Read the model definition and answer for the solid it produces. Units are mm, in the model's axes. Face numbers are marked on the shaded views. A direction names the side the tool comes from. Coordinates: 2 decimals unless noted, no trailing zeros. Loops run counter-clockwise (first coordinate to the right, second up) from the corner with the lowest first, then second, coordinate; pieces in that order, holes last.
Q1. Flat-ended cylindrical pins translate along their axes: P1, Ø5, axis at y = 14.5, z = -1, coming from the +X side; P2, Ø1.5, axis at x = -4.5, y = 10, coming from the -Z side; P3, Ø3, axis at y = 15.5, z = -11.5, coming from the -X side; P4, Ø10, axis at x = -3.5, y = 11.5, coming from the +Z side. Find the tip coordinate at first contact, or state that the pin passes through.
Q2. Straight lines are drawn through the part: line 1 (X direction, y = 2.6, z = -16); line 2 (Y direction, x = -4.5, z = -4.5); line 3 (Y direction, x = 4.25, z = -10). For each, find the intervals that lie inside material, in ascending order.
Q3. The mould has two halves that part along X. Classify the marked faces 4, 5, 6 and 7: pulls with the +X half, pulls with the -X half, needs draft (parallel to the pull), parting line crosses it, or undercut.
Q4. Section A-A (z = -16) is taken. Give the vertices of the cut face in (x, y), then the cut area to 3 significant figures.
Q5. Section B-B (y = 18.5) is taken. Give the vertices of the cut face in (x, z).
Q6. Which of the six approach directions +Z, -Z, +X, -X, +Y, -Y give full straight-line access (tool end or side, diameter ignored) to the marked faces 1, 2 and 3?
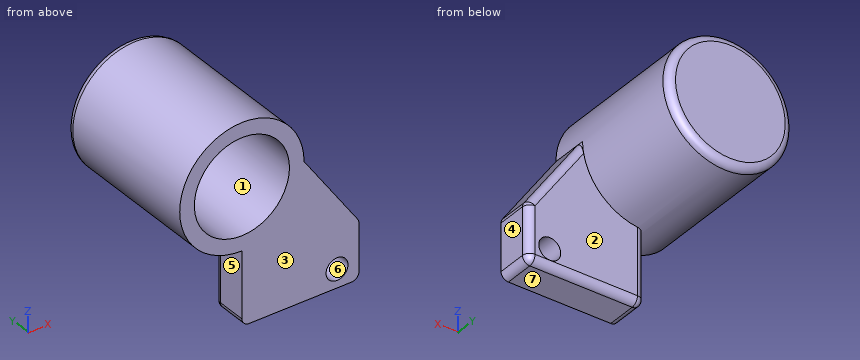
from build123d import *

# Parameters (mm, degrees)
SALIENTE_EXTRUIR1_START = -5
CROQUIS2_R              = 1.5
SALIENTE_EXTRUIR1_DEPTH = 5
REDONDEO1_R             = 1


with BuildPart() as part:
    # Croquis1 → Revolución1 (revolve)
    with BuildSketch(Plane.XY, mode=Mode.PRIVATE) as revoluci_n1_sk:
        Polygon((0, 19), (-6.5, 19), (-6.5, 0), (-8.5, 0), (-8.5, 21), (0, 21), align=None)
    revolve(revoluci_n1_sk.sketch.rotate(Axis((0, 0, 0), (0, 1, 0)), 270), axis=Axis((0, 0, 0), (0, 1, 0)))

    # Croquis2 → Saliente-Extruir1 (add)
    with BuildSketch(Plane.XZ.offset(SALIENTE_EXTRUIR1_START)):
        with BuildLine():
            Line((10, -18.5), (16, -18.5))
            Line((16, -18.5), (16, -10.75))
            Line((16, -10.75), (8.5, 0))
            ThreePointArc((8.5, 0), (6.01040764, -6.01040764), (0, -8.5))
            Line((0, -8.5), (0, -18.5))
            Line((0, -18.5), (10, -18.5))
        make_face()
        with Locations(Location((13, -16, 0), (0, 0, 270))):
            Circle(CROQUIS2_R, mode=Mode.SUBTRACT)
    extrude(amount=SALIENTE_EXTRUIR1_DEPTH)

    # Redondeo1
    # the kernel refuses this fillet: 1 mm, written as the material it takes off along each edge
    with BuildSketch(Plane(origin=(15, 4, -11.064363564), x_dir=(0.8201269543011832, 0, 0.5721815960240815), z_dir=(0, 1, 0))) as redondeo1_piece_1_section:
        Polygon((0, 0), (REDONDEO1_R, 0), (REDONDEO1_R, REDONDEO1_R * 0.314363563856), (REDONDEO1_R * 0.820126954301, REDONDEO1_R * 0.572181596024), align=None)
    redondeo1_piece_1 = extrude(amount=REDONDEO1_R, mode=Mode.PRIVATE)
    redondeo1_piece_1 = redondeo1_piece_1 - Plane(origin=(15, 4, -11.064363564), x_dir=(-0.9539724719039809, 0, -0.29989418608804086), z_dir=(0, 1, 0)) * Sphere(REDONDEO1_R, mode=Mode.PRIVATE)
    add(redondeo1_piece_1, mode=Mode.SUBTRACT)
    with BuildSketch(Plane(origin=(15, 4, -17.5), x_dir=(1, 0, 0), z_dir=(0, 0, -1))) as redondeo1_piece_2_section:
        Polygon((0, 0), (REDONDEO1_R, 0), (REDONDEO1_R, -REDONDEO1_R), (0, -REDONDEO1_R), align=None)
    redondeo1_piece_2 = extrude(amount=REDONDEO1_R, mode=Mode.PRIVATE)
    redondeo1_piece_2 = redondeo1_piece_2 - Plane(origin=(15, 4, -17.5), x_dir=(-0.7071067811865475, -0.7071067811865475, 0), z_dir=(0, 0, -1)) * Sphere(REDONDEO1_R, mode=Mode.PRIVATE)
    add(redondeo1_piece_2, mode=Mode.SUBTRACT)
    with BuildSketch(Plane(origin=(1, 4, -17.5), x_dir=(-1, 0, 0), z_dir=(0, 0, -1))) as redondeo1_piece_3_section:
        Polygon((0, 0), (REDONDEO1_R, 0), (REDONDEO1_R, REDONDEO1_R), (0, REDONDEO1_R), align=None)
    redondeo1_piece_3 = extrude(amount=REDONDEO1_R, mode=Mode.PRIVATE)
    redondeo1_piece_3 = redondeo1_piece_3 - Plane(origin=(1, 4, -17.5), x_dir=(0.7071067811865475, -0.7071067811865475, 0), z_dir=(0, 0, -1)) * Sphere(REDONDEO1_R, mode=Mode.PRIVATE)
    add(redondeo1_piece_3, mode=Mode.SUBTRACT)
    with BuildSketch(Plane(origin=(15.820126954, 5, -10.492181968), x_dir=(-0.8201269543011831, 0, -0.5721815960240815), z_dir=(-0.5721815960240815, 0, 0.8201269543011832))) as redondeo1_piece_4_section:
        with BuildLine():
            CenterArc((REDONDEO1_R, REDONDEO1_R), REDONDEO1_R, 180, 90)
            Line((0, REDONDEO1_R), (0, 0))
            Line((0, 0), (REDONDEO1_R, 0))
        make_face()
    redondeo1_piece_4 = extrude(amount=15.293363165, mode=Mode.PRIVATE)
    redondeo1_piece_4 = redondeo1_piece_4 - Plane(origin=(0, 4.770801137, 0), x_dir=(0, 0, -1), z_dir=(0, 1, 0)) * Cylinder(8.5, 35, mode=Mode.PRIVATE)
    add(redondeo1_piece_4, mode=Mode.SUBTRACT)
    with BuildSketch(Plane(origin=(16, 5, -17.5), x_dir=(-1, 0, 0), z_dir=(0, 0, 1))) as redondeo1_piece_5:
        with BuildLine():
            CenterArc((REDONDEO1_R, REDONDEO1_R), REDONDEO1_R, 180, 90)
            Line((0, REDONDEO1_R), (0, 0))
            Line((0, 0), (REDONDEO1_R, 0))
        make_face()
    extrude(amount=6.435636436, mode=Mode.SUBTRACT)
    with BuildSketch(Plane(origin=(16, 4, -10.75), x_dir=(-0.5721815960240826, 0, 0.8201269543011824), z_dir=(0, -1, 0))) as redondeo1_piece_6:
        with BuildLine():
            CenterArc((REDONDEO1_R * 0.314363563856, REDONDEO1_R), REDONDEO1_R, 235.097504384, 34.902495616)
            Line((-REDONDEO1_R * 0.257818032168, REDONDEO1_R * 0.179873045699), (0, 0))
            Line((0, 0), (REDONDEO1_R * 0.314363563856, 0))
        make_face()
    extrude(amount=4.78590891, mode=Mode.SUBTRACT)
    with BuildSketch(Plane(origin=(1, 5, -18.5), x_dir=(0, 0, 1), z_dir=(1, 0, 0))) as redondeo1_piece_7:
        with BuildLine():
            CenterArc((REDONDEO1_R, REDONDEO1_R), REDONDEO1_R, 180, 90)
            Line((0, REDONDEO1_R), (0, 0))
            Line((0, 0), (REDONDEO1_R, 0))
        make_face()
    extrude(amount=14, mode=Mode.SUBTRACT)
    with BuildSketch(Plane(origin=(16, 4, -18.5), x_dir=(-1, 0, 0), z_dir=(0, -1, 0)), Plane(origin=(0, 4, -18.5), x_dir=(0, 0, 1), z_dir=(0, -1, 0))) as redondeo1_piece_8:
        with BuildLine():
            CenterArc((REDONDEO1_R, -REDONDEO1_R), REDONDEO1_R, 90, 90)
            Line((0, -REDONDEO1_R), (0, 0))
            Line((0, 0), (REDONDEO1_R, 0))
        make_face()
    extrude(amount=6.5, mode=Mode.SUBTRACT)
    with BuildSketch(Plane(origin=(0, 5, -6), x_dir=(0, -1, 0), z_dir=(0, 0, -1))) as redondeo1_piece_9_section:
        with BuildLine():
            CenterArc((REDONDEO1_R, -REDONDEO1_R), REDONDEO1_R, 90, 90)
            Line((0, -REDONDEO1_R), (0, 0))
            Line((0, 0), (REDONDEO1_R, 0))
        make_face()
    redondeo1_piece_9 = extrude(amount=11.5, mode=Mode.PRIVATE)
    redondeo1_piece_9 = redondeo1_piece_9 - Plane(origin=(0, 4.773710582, 0), x_dir=(0, 0, -1), z_dir=(0, 1, 0)) * Cylinder(8.5, 27, mode=Mode.PRIVATE)
    add(redondeo1_piece_9, mode=Mode.SUBTRACT)
    with BuildSketch(Plane(origin=(0, 21, 0), x_dir=(0, 0, -1), z_dir=(1, 0, 0))) as redondeo1_piece_10:
        with BuildLine():
            CenterArc((8.5 - REDONDEO1_R, -REDONDEO1_R), REDONDEO1_R, 0, 90)
            Line((8.5 - REDONDEO1_R, 0), (8.5, 0))
            Line((8.5, 0), (8.5, -REDONDEO1_R))
        make_face()
    revolve(axis=Axis((0, 21, 0), (0, 1, 0)), mode=Mode.SUBTRACT)


solid = part.part
Numbers:
1. P1: stops at x = 8.5
1. P2: stops at z = -7.63
1. P3: passes through
1. P4: stops at z = 8.5
2. line 1: x = 0 to 11.5, 14.5 to 16
2. line 2: y = 19 to 21
2. line 3: y = 0 to 5
3. face 4: pulls with the +X half
3. face 5: pulls with the -X half
3. face 6: undercut
3. face 7: needs draft
4. outline: (0, 0) - (11.5, 0) - (11.5, 5) - (1, 5) arc R1 ccw to (0, 4) - close; (14.5, 0) - (16, 0) - (16, 4) arc R1 ccw to (15, 5) - (14.5, 5) - close
4. area: 64.6 mm2
5. outline: circle Ø17 at (0, 0); hole circle Ø13 at (0, 0)
6. face 1: -Y
6. face 2: -Z, +X, +Y
6. face 3: +Z, -Z, +X, -X, -Y
